Check sheet for the drawn part. Datum: minimum x, y, z corner. Units: mm. A direction names the side the tool comes from. Give positions to 0.01 mm unless a question says otherwise; leave off trailing zeros. Write each loop counter-clockwise with the first axis right and the second up, starting at its lowest first coordinate (ties: lowest second). Pieces come first, ordered by that corner, then holes. Notation, with made-up numbers: (67, 56.5) - (107, 56.5) arc R22 cw to (107, 63.5) - close; hole circle Ø6 at (-1.75, 59.25). An arc over 180 degrees is marked (long way). One line per question, with ' | ' between items. Start each with the question number.
Q1. Section check D-D on z = 17.5. Record the boundary of the cut face in (x, y).
Q2. Set-up check for the marked faces 1 and 2: record each of +Z, -Z, +X, -X, +Y, -Y from which the full face is reachable in a straight line by a thin tool's end or side.
Q3. Section check A-A on z = 11. Record the boundary of the cut face in (x, y), and give its area (4 significant figures).
Q4. Section check B-B on y = 30. Record the boundary of the cut face in (x, z), and give its area (3 significant figures).
Q5. Thickness scan on L1, parallel to X at y = 38, z = 13; L2, parallel to Y at x = 57, z = 17.5; L3, parallel to Z at x = 63, y = 30. Record the ranges inside material, lowest first. Write a range as [from, to].
Q6. Gauge pin test, flat ends, axial feed: P1, Ø7.5, axis at y = 52, z = 17, coming from the +X side; P2, Ø12, axis at x = 21, y = 35, coming from the +Z side; P3, Ø5, axis at y = 52.5, z = 10, coming from the +X side. Record the tip position at first contact, or that the pin passes through.
Q7. Release check for a two-part mould opening along X. For the marked faces 3, 4, 5 and 6 record: +X half, -X half, draft (parallel to the pull), parting line (faces both ways), or undercut.
Q8. Section check C-C on x = 64. Record the boundary of the cut face in (y, z).
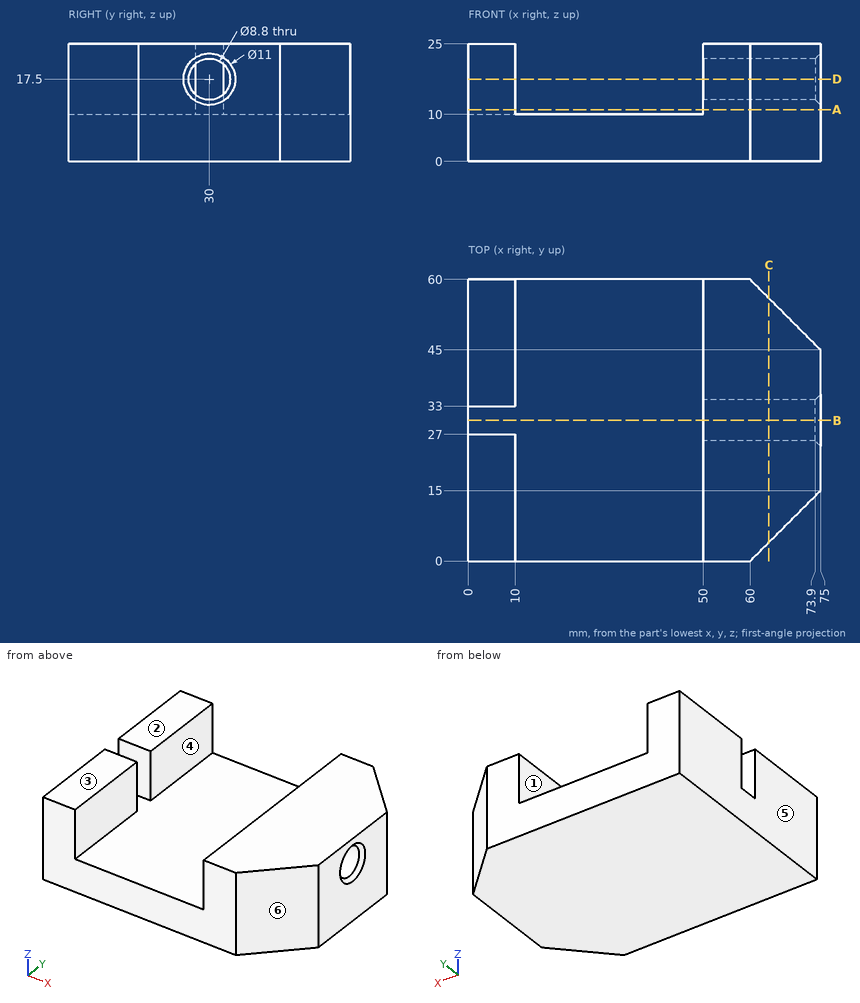
Working result:
1) outline: (0, 0) - (10, 0) - (10, 27) - (0, 27) - close; (0, 33) - (10, 33) - (10, 60) - (0, 60) - close; (50, 0) - (60, 0) - (75, 15) - (75, 24.5) - (73.9, 25.6) - (50, 25.6) - close; (50, 34.4) - (73.9, 34.4) - (75, 35.5) - (75, 45) - (60, 60) - (50, 60) - close
2) face 1: +Z, +Y, -Y | face 2: +Z, +X, -X, +Y, -Y
3) outline: (0, 0) - (10, 0) - (10, 27) - (0, 27) - close; (0, 33) - (10, 33) - (10, 60) - (0, 60) - close; (50, 0) - (60, 0) - (75, 15) - (75, 45) - (60, 60) - (50, 60) - close | area: 1,815 mm2
4) outline: (0, 0) - (75, 0) - (75, 12) - (73.9, 13.1) - (50, 13.1) - (50, 10) - (0, 10) - close; (50, 21.9) - (73.9, 21.9) - (75, 23) - (75, 25) - (50, 25) - close | area: 904 mm2
5) L1: x = [0, 10], [50, 75] | L2: y = [0, 25.6], [34.4, 60] | L3: z = [0, 13.1], [21.9, 25]
6) P1: stops at x = 71.75 | P2: stops at z = 10 | P3: stops at x = 70
7) face 3: draft | face 4: undercut | face 5: -X half | face 6: +X half
8) outline: (4, 0) - (56, 0) - (56, 25) - (4, 25) - close; hole circle Ø8.8 at (30, 17.5)
